Design review of the part built by this model. Coordinates are the model's own, in mm. A direction names the side the tool comes from. Round coordinates to 2 decimals unless told otherwise and drop trailing zeros. Order: outer loops, then holes, each group sorted by start corner. A loop starts at its lowest first (then second) coordinate and runs counter-clockwise, first axis right, second up. Notation, with made-up numbers: M 77.5,-13.5 L 130.5,-13.5 A20 ccw 130.5,-2.5 Z; hole C 85,39 d11. An arc over 180 degrees is marked long. Use a Markdown table: item, result. Add a question column.
(1) To check wall thickness, follow probe 1 along Y at (x, z) = (67.5, 7); probe 2 along X at (y, z) = (92.5, 9.5); probe 3 along X at (y, z) = (-97, 8.75). State the ranges of each line that lie inside material, in increasing order. Write a range as from..to.
(2) For pin 1 (1.1 mm diameter, centred on x = -64, y = -89, fed in from +Z), flat-tipped, find the tip position at first contact; note if it passes through.
(3) The part is to be moulded in two halves that separate along X. For faces 4 (the face through (68.53, 87.863, 2.712)), 5 (the face through (-78, 8, 3)), say which applies: released by +X, released by -X, zero draft, split by the parting line, or undercut.
(4) Take a section at A-A (y = -4.5). Write out the cut boundary in (x, z), then the cut area to 3 significant figures.
(5) Take a section at B-B (x = 27). Write out the cut boundary in (y, z), then the cut area to 3 significant figures.
(6) Take a section at C-C (z = 9). Count the separate pieces of the cut face and the enclosed holes in it, then the cut area to 3 significant figures.
(7) Machinability: for faces 1 (the face through (70, 95, 5.5)), 2 (the face through (66, -95, 12)), 3 (the face through (69.297, -94.165, 8.704)), which of the approach directions +Z, -Z, +X, -X, +Y, -Y give a long, thin tool a straight path to every point of the face, cutting with its end or side? Answer none if there is none.
Autodesk Inventor part; units mm, degrees
ref_plane "YZ Plane" through (0, 0, 0) normal (1, 0, 0) x (0, 1, 0)
ref_plane "XZ Plane" through (0, 0, 0) normal (0, 1, 0) x (-1, 0, 0)
ref_plane "XY Plane" through (0, 0, 0) normal (0, 0, 1) x (1, 0, 0)
sketch "Boceto1" plane through (0, 0, 0) normal (0, 0, 1) x (1, 0, 0)
  line L0 (-83, -108.2) -> (83, -108.2)
  line L1 (83, -108.2) -> (83, 108.2)
  line L2 (83, 108.2) -> (-83, 108.2)
  line L3 (-83, 108.2) -> (-83, -108.2)
  line L4 (-83, -108.2) -> (83, 108.2) construction
  line L5 (83, -108.2) -> (-83, 108.2) construction
  point P0 (0, 0)
  dimension "d0" = 166
  dimension "d1" = 216.4
extrude "Extrusión1" add sketch "Boceto1" along normal blind 15
sketch "Boceto2" plane through (0, 0, 15) normal (0, 0, 1) x (1, 0, 0)
  line L0 (80.75, -105.95) -> (-80.75, -105.95)
  line L1 (-80.75, -105.95) -> (-80.75, 105.95)
  line L2 (80.75, 105.95) -> (-80.75, 105.95)
  line L3 (80.75, 105.95) -> (80.75, -105.95)
  line L4 (-83, 108.2) -> (83, 108.2)
  line L5 (83, 108.2) -> (83, -108.2)
  line L6 (83, -108.2) -> (-83, -108.2)
  line L7 (-83, -108.2) -> (-83, 108.2)
  point P0 (0, 0)
extrude "Extrusión2" cut sketch "Boceto2" against normal blind 12 contours L0 L1 L2 L3
sketch "Boceto3" plane through (0, 0, 3) normal (0, 0, 1) x (1, 0, 0)
  line L0 (-67.5, -92.5) -> (67.5, -92.5)
  line L1 (67.5, -92.5) -> (67.5, 92.5)
  line L2 (67.5, 92.5) -> (-67.5, 92.5)
  line L3 (-67.5, 92.5) -> (-67.5, -92.5)
  line L4 (-62.5, 87.5) -> (-72.5, 87.5)
  line L5 (-72.5, 87.5) -> (-72.5, 97.5)
  line L6 (-72.5, 97.5) -> (-62.5, 97.5)
  line L7 (-62.5, 97.5) -> (-62.5, 87.5)
  line L8 (-62.5, 87.5) -> (-72.5, 97.5) construction
  line L9 (-72.5, 87.5) -> (-62.5, 97.5) construction
  line L10 (72.5, 87.5) -> (62.5, 87.5)
  line L11 (62.5, 87.5) -> (62.5, 97.5)
  line L12 (62.5, 97.5) -> (72.5, 97.5)
  line L13 (72.5, 97.5) -> (72.5, 87.5)
  line L14 (72.5, 87.5) -> (62.5, 97.5) construction
  line L15 (62.5, 87.5) -> (72.5, 97.5) construction
  line L16 (72.5, -97.5) -> (62.5, -97.5)
  line L17 (62.5, -97.5) -> (62.5, -87.5)
  line L18 (62.5, -87.5) -> (72.5, -87.5)
  line L19 (72.5, -87.5) -> (72.5, -97.5)
  line L20 (72.5, -97.5) -> (62.5, -87.5) construction
  line L21 (62.5, -97.5) -> (72.5, -87.5) construction
  line L22 (-62.5, -97.5) -> (-72.5, -97.5)
  line L23 (-72.5, -97.5) -> (-72.5, -87.5)
  line L24 (-72.5, -87.5) -> (-62.5, -87.5)
  line L25 (-62.5, -87.5) -> (-62.5, -97.5)
  line L26 (-62.5, -97.5) -> (-72.5, -87.5) construction
  line L27 (-72.5, -97.5) -> (-62.5, -87.5) construction
  point P0 (0, 0)
  dimension "d12" = 135
  dimension "d13" = 185
  dimension "d14" = 10
  dimension "d15" = 10
  dimension "d16" = 10
  dimension "d17" = 10
  dimension "d18" = 10
  dimension "d19" = 10
  dimension "d20" = 10
  dimension "d21" = 10
extrude "Extrusión3" add sketch "Boceto3" along normal blind 9 contours L3 L24 L25 L0 | L0 L25 L22 L23 L24 L3 | L17 L18 L1 L0 | L0 L1 L18 L19 L16 L17 | L4 L5 L6 L7 L2 L3 | L3 L2 L7 L4 | L10 L11 L2 L1 | L1 L2 L11 L12 L13 L10
sketch "Boceto4" plane through (0, 0, 0) normal (0, 0, -1) x (-1, 0, 0)
  line L0 (72.5, -97.5) -> (72.5, -87.5)
  line L1 (72.5, -87.5) -> (62.5, -87.5)
  line L2 (62.5, -87.5) -> (62.5, -97.5)
  line L3 (62.5, -97.5) -> (72.5, -97.5)
  line L4 (-62.5, 87.5) -> (-62.5, 97.5)
  line L5 (-62.5, 97.5) -> (-72.5, 97.5)
  line L6 (-72.5, 97.5) -> (-72.5, 87.5)
  line L7 (-72.5, 87.5) -> (-62.5, 87.5)
  line L8 (72.5, 87.5) -> (72.5, 97.5)
  line L9 (72.5, 97.5) -> (62.5, 97.5)
  line L10 (62.5, 97.5) -> (62.5, 87.5)
  line L11 (62.5, 87.5) -> (72.5, 87.5)
  line L12 (-62.5, -97.5) -> (-62.5, -87.5)
  line L13 (-62.5, -87.5) -> (-72.5, -87.5)
  line L14 (-72.5, -87.5) -> (-72.5, -97.5)
  line L15 (-72.5, -97.5) -> (-62.5, -97.5)
  line L16 (80.75, -105.95) -> (80.75, 105.95)
  line L17 (-80.75, -105.95) -> (80.75, -105.95)
  line L18 (-80.75, 105.95) -> (-80.75, -105.95)
  line L19 (80.75, 105.95) -> (-80.75, 105.95)
  line L20 (-67.5, -92.5) -> (-67.5, 92.5)
  line L21 (67.5, 92.5) -> (67.5, -92.5)
  line L22 (-67.5, 92.5) -> (67.5, 92.5)
  line L23 (67.5, -92.5) -> (-67.5, -92.5)
  circle A0 centre (-67.5, 92.5) radius 4.75
  circle A1 centre (67.5, 92.5) radius 4.75
  circle A2 centre (67.5, -92.5) radius 4.75
  circle A3 centre (-67.5, -92.5) radius 4.75
  point P0 (0, 0)
  dimension "d24" = 9.5
  dimension "d25" = 9.5
  dimension "d26" = 9.5
  dimension "d27" = 9.5
extrude "Extrusión4" cut sketch "Boceto4" against normal blind 5.5 contours A2 L23 L21 | L21 L23 A2 | A1 L22 L21 | L21 L22 A1 | A3 L20 L23 | L23 L20 A3 | A0 L20 L22 | L22 L20 A0
sketch "Boceto5" plane through (67.5, 92.5, 5.5) normal (0, 0, -1) x (-1, 0, 0)
  arc A0 (2.2886, -0.8744) -> (0.8744, -2.2886) centre (0, 0) ccw
  line L0 (0, 0) -> (4.75, 0) construction
  line L1 (1.6679, -3.0821) -> (2.5764, -3.9906)
  line L2 (1.6679, -3.0821) -> (0.8744, -2.2886)
  line L3 (2.2886, -0.8744) -> (3.9906, -2.5764)
  arc A1 (2.5764, -3.9906) -> (3.9906, -2.5764) centre (0, 0) ccw
  line L4 (135, -185) -> (0, -185)
  arc A2 (134.1256, -2.2886) -> (132.7114, -0.8744) centre (135, 0) ccw
  line L5 (131.9179, -1.6679) -> (131.0094, -2.5764)
  line L6 (131.9179, -1.6679) -> (132.7114, -0.8744)
  line L7 (134.1256, -2.2886) -> (132.4236, -3.9906)
  arc A3 (131.0094, -2.5764) -> (132.4236, -3.9906) centre (135, 0) ccw
  arc A4 (132.7114, -184.1256) -> (134.1256, -182.7114) centre (135, -185) ccw
  line L8 (133.3321, -181.9179) -> (132.4236, -181.0094)
  line L9 (133.3321, -181.9179) -> (134.1256, -182.7114)
  line L10 (132.7114, -184.1256) -> (131.0094, -182.4236)
  arc A5 (132.4236, -181.0094) -> (131.0094, -182.4236) centre (135, -185) ccw
  arc A6 (0.8744, -182.7114) -> (2.2886, -184.1256) centre (0, -185) ccw
  line L11 (3.0821, -183.3321) -> (3.9906, -182.4236)
  line L12 (3.0821, -183.3321) -> (2.2886, -184.1256)
  line L13 (0.8744, -182.7114) -> (2.5764, -181.0094)
  arc A7 (3.9906, -182.4236) -> (2.5764, -181.0094) centre (0, -185) ccw
  point P0 (67.5, -92.5)
  dimension "d30" = 4.9
  dimension "d36" = 4.9
  dimension "d37" = 4.9
  dimension "d38" = 4.9
extrude "Extrusión5" cut sketch "Boceto5" against normal blind 10
sketch "Boceto6" plane through (0, 0, 3) normal (0, 0, 1) x (1, 0, 0)
  line L0 (62.5, -87.5) -> (62.5, -97.5)
  line L1 (72.5, -87.5) -> (62.5, -87.5)
  line L2 (-62.5, -97.5) -> (-62.5, -87.5)
  line L3 (-57.5, -97.5) -> (-57.5, -100.837)
  line L4 (-57.5, -100.837) -> (57.5, -100.837)
  line L5 (57.5, -100.837) -> (57.5, -82.5)
  line L6 (75.7581, -82.5) -> (57.5, -82.5)
  line L7 (-57.5, -100.837) -> (-57.5, -82.5)
  line L8 (-80.75, -105.95) -> (-80.75, 105.95)
  line L9 (75.7581, 82.5) -> (57.5081, 82.4907)
  line L10 (-80.75, 105.95) -> (80.75, 105.95)
  line L11 (57.5081, 105.95) -> (57.5081, 105.95)
  line L12 (57.5, -105.837) -> (57.5, -105.95)
  arc A0 (57.5, -105.837) -> (62.5, -100.837) centre (57.5, -100.837) ccw
  line L13 (62.5, -100.837) -> (62.5, -87.5)
  line L14 (72.5, -82.5) -> (75.7581, -82.5)
  line L15 (62.5, -87.5) -> (75.75, -87.5)
  line L16 (75.7581, -82.5) -> (75.7581, 82.5)
  arc A1 (75.8451, -87.4992) -> (80.7581, -82.5) centre (75.7581, -82.5) ccw
  arc A2 (80.7581, 82.5082) -> (75.75, 87.5) centre (75.7581, 82.5) ccw
  line L17 (62.5, 87.5) -> (72.5, 87.5)
  line L18 (75.75, 87.5) -> (62.5, 87.5)
  line L19 (62.5, 87.5) -> (62.5, 101.2352)
  line L20 (62.5, 97.5) -> (62.5, 87.5)
  arc A3 (62.5, 101.2352) -> (57.5081, 105.95) centre (57.5081, 100.95) ccw
  line L21 (57.5081, 82.4907) -> (57.5081, 100.95)
  line L22 (57.5081, 105.95) -> (57.5081, 105.95)
  arc A4 (-57.5, 105.95) -> (-62.5, 100.95) centre (-57.5, 100.95) ccw
  line L23 (-62.5, 87.5) -> (-62.5, 97.5)
  line L24 (-62.5, 100.95) -> (-62.5, 87.5)
  line L25 (-72.5, 97.5) -> (-72.5, 87.5)
  line L26 (-57.5, 82.5) -> (-57.5, 100.95)
  line L27 (-75.75, 82.5) -> (-75.75, -82.5)
  arc A5 (-75.75, 87.5) -> (-80.75, 82.5) centre (-75.75, 82.5) ccw
  line L28 (-75.75, 82.5) -> (-57.5, 82.5)
  line L29 (-62.5, 87.5) -> (-75.75, 87.5)
  line L30 (-62.5, -87.5) -> (-72.5, -87.5)
  arc A6 (-80.75, -82.5) -> (-75.75, -87.5) centre (-75.75, -82.5) ccw
  arc A7 (-62.5, -100.837) -> (-57.5, -105.837) centre (-57.5, -100.837) ccw
  line L31 (-75.75, -87.5) -> (-62.5, -87.5)
  line L32 (-62.5, -100.837) -> (-62.5, -87.5)
  line L33 (57.5, -105.837) -> (-57.5, -105.837)
  line L34 (80.75, -105.95) -> (-80.75, -105.95)
  line L35 (-80.75, -82.5) -> (-80.75, 82.5)
  line L36 (-57.5, 105.95) -> (57.5081, 105.95)
  line L37 (80.7581, 82.5082) -> (80.7581, -82.5)
  line L38 (-75.75, -82.5) -> (-57.5, -82.5)
  line L39 (57.5081, 100.95) -> (-57.5, 100.95)
  point P0 (0, 0)
  dimension "d52" = 5
extrude "Extrusión6" cut sketch "Boceto6" against normal blind 10 contours L7 L38 L27 L28 L26 L39 L21 L9 L16 L6 L5 L4 L3
properties part number "TestTapa_v0"
Verdict:
| question | item | result |
|---|---|---|
| 1 | probe 1 | y = -108.2..-105.95, -97.5..-94.95, -90.05..-87.5, 87.5..90.05, 94.95..97.5, 105.95..108.2 |
| 1 | probe 2 | x = -83..-80.75, -72.5..-69.95, -65.05..-62.5, 62.5..65.05, 69.95..72.5, 80.75..83 |
| 1 | probe 3 | x = -83..-80.75, -72.5..-62.5, 62.5..72.5, 80.75..83 |
| 2 | pin 1 | stops at z = 12 |
| 3 | face 4 | undercut |
| 3 | face 5 | undercut |
| 4 | outline | M -83,0 L -75.75,0 L -75.75,3 L -80.75,3 L -80.75,15 L -83,15 Z; M 75.76,0 L 83,0 L 83,15 L 80.75,15 L 80.75,3 L 75.76,3 Z |
| 4 | area | 97.5 mm^2 |
| 5 | outline | M -108.2,0 L -100.84,0 L -100.84,3 L -105.95,3 L -105.95,15 L -108.2,15 Z; M 100.95,0 L 108.2,0 L 108.2,15 L 105.95,15 L 105.95,3 L 100.95,3 Z |
| 5 | area | 97.8 mm^2 |
| 6 | separate pieces | 5 |
| 6 | enclosed holes | 5 |
| 6 | area | 2,010 mm^2 |
| 7 | face 1 | -Z |
| 7 | face 2 | +Z |
| 7 | face 3 | +Z, -Z |
